Design review of the part built by this model. Coordinates are the model's own, in mm. A direction names the side the tool comes from. Round coordinates to 2 decimals unless told otherwise and drop trailing zeros. Write each loop counter-clockwise with the first axis right and the second up, starting at its lowest first coordinate (ties: lowest second). Pieces come first, ordered by that corner, then holes. Notation, with made-up numbers: (68.5, 57) -> (84.5, 57) arc R16 cw to (84.5, 82) -> close; hole circle Ø4 at (24.25, -21). An arc over 180 degrees is marked (long way). Write item = value, one per line. Start each with the question number.
Item 1: Machinability: for faces 4 (the flat face through (12, 5.359, 0)), 5 (the flat face through (1, 14.275, 3)), 6 (the flat face through (11.836, 6, 0)), which of the approach directions +Z, -Z, +X, -X, +Y, -Y give a long, thin tool a straight path to every point of the face, cutting with its end or side? Answer none if there is none.
Item 2: To check wall thickness, follow L1, parallel to Z at x = 12.5, y = 5.5; L2, parallel to Y at x = 7, z = -2.5; L3, parallel to X at y = 4.75, z = 4.25. State the ranges of each line that lie inside material, in increasing order.
Item 3: Add section D-D, the plane y = 15.5. State the section outline as (x, z) points, then the cut area to 3 significant figures.
Item 4: Add section B-B, the plane z = 0. State the section outline as (x, y) points, then the cut area to 3 significant figures.
Item 5: Mouldability with a two-part tool opening along Z and no side actions: class faces 1 (the flat face through (14, 5.613, 0)), 2 (the flat face through (0, 16.027, 0)), 3 (the cylindrical face through (5.16, 7.58, -1.63)) as released by +Z, released by -Z, zero draft, split by the parting line, or undercut.
Item 6: Add section A-A, the plane x = 10.5. State the section outline as (y, z) points, then the cut area to 3 significant figures.
Item 7: Add section C-C, the plane y = 4. State the section outline as (x, z) points, then the cut area to 3 significant figures.
Item 8: For pin 1 Ø5 at (x, z) = (12, -1.5) entering from +Y; pin 2 Ø2 at (y, z) = (13, 5.5) entering from +X; pin 3 Ø5 at (y, z) = (3.5, 3.5) entering from -X; pin 4 Ø1.1 at (x, z) = (13.5, 6) entering from -Y, all flat-tipped, find the tip position at first contact; note any pin that passes through.
from build123d import *

# Parameters (mm, degrees)
SKETCH1_R           = 8.1534
BOSS_EXTRUDE1_DEPTH = 5.6134
BOSS_EXTRUDE2_DEPTH = 1.27
BOSS_EXTRUDE3_DEPTH = 0.254
SKETCH4_R           = 5.4102
BOSS_EXTRUDE4_DEPTH = 0.889
SKETCH5_R           = 3.3655
BOSS_EXTRUDE5_DEPTH = 6.2484
SKETCH6_R           = 2.9591
BOSS_EXTRUDE6_DEPTH = 8.509
SKETCH7_W           = 8.77263503
SKETCH7_H           = 1.27
CUT_EXTRUDE1_DEPTH  = 6.7564
BOSS_EXTRUDE7_DEPTH = 0.254
LPATTERN1_COUNT     = 2
LPATTERN1_PITCH     = 5.207
LPATTERN2_COUNT     = 2
LPATTERN2_PITCH     = 5.207
FILLET1_R           = 0.762


with BuildPart() as part:
    # Sketch1 → Boss-Extrude1 (new body)
    with BuildSketch(Plane(origin=(0, 0, 0), x_dir=(1, 0, 0), z_dir=(0, 1, 0))):
        Circle(SKETCH1_R)
    extrude(amount=BOSS_EXTRUDE1_DEPTH)

    # Sketch2 → Boss-Extrude2 (add)
    with BuildSketch(Plane(origin=(0, 5.6134, 0), x_dir=(1, 0, 0), z_dir=(0, 1, 0))):
        with BuildLine():
            Line((0, 8.1534), (11.8364, 8.1534))
            Line((11.8364, 8.1534), (11.8364, -8.1534))
            Line((11.8364, -8.1534), (0, -8.1534))
            ThreePointArc((0, -8.1534), (-8.1534, 0), (0, 8.1534))
        make_face()
    extrude(amount=BOSS_EXTRUDE2_DEPTH)

    # Sketch3 → Boss-Extrude3 (add)
    with BuildSketch(Plane(origin=(0, 6.8834, 0), x_dir=(1, 0, 0), z_dir=(0, 1, 0))):
        with BuildLine():
            Line((-5.4737, 5.301227057), (-5.4737, -5.301227057))
            ThreePointArc((-5.4737, -5.301227057), (0, -7.62), (5.4737, -5.301227057))
            Line((5.4737, -5.301227057), (5.4737, 5.301227057))
            ThreePointArc((5.4737, 5.301227057), (0, 7.62), (-5.4737, 5.301227057))
        make_face()
    extrude(amount=BOSS_EXTRUDE3_DEPTH)

    # Sketch4 → Boss-Extrude4 (add)
    with BuildSketch(Plane(origin=(0, 7.1374, 0), x_dir=(1, 0, 0), z_dir=(0, 1, 0))):
        Circle(SKETCH4_R)
    extrude(amount=BOSS_EXTRUDE4_DEPTH)

    # Sketch5 → Boss-Extrude5 (add)
    with BuildSketch(Plane(origin=(0, 8.0264, 0), x_dir=(1, 0, 0), z_dir=(0, 1, 0))):
        Circle(SKETCH5_R)
    extrude(amount=BOSS_EXTRUDE5_DEPTH)

    # Sketch6 → Boss-Extrude6 (add)
    with BuildSketch(Plane(origin=(0, 14.2748, 0), x_dir=(1, 0, 0), z_dir=(0, 1, 0))):
        Circle(SKETCH6_R)
    extrude(amount=BOSS_EXTRUDE6_DEPTH)

    # Sketch7 → Cut-Extrude1 (cut)
    with BuildSketch(Plane(origin=(0, 22.7838, 0), x_dir=(1, 0, 0), z_dir=(0, 1, 0))):
        Rectangle(SKETCH7_W, SKETCH7_H)
    extrude(amount=-CUT_EXTRUDE1_DEPTH, mode=Mode.SUBTRACT)

    # Sketch8 → Boss-Extrude7 (add)
    with BuildSketch(Plane.XZ.offset(-5.6134)):
        Polygon((8.350699667, 1.7526), (12.8524, 1.7526), (12.8524, 0.4826), (16.5862, 0.4826), (16.5862, -0.4826), (12.8524, -0.4826), (12.8524, -1.7526), (8.350699667, -1.7526), align=None)
    boss_extrude7 = extrude(amount=BOSS_EXTRUDE7_DEPTH)

    # LPattern1: Boss-Extrude7 ×2
    with Locations(*[(0, 0, -i * LPATTERN1_PITCH) for i in range(1, LPATTERN1_COUNT)]):
        add(boss_extrude7)

    # LPattern2: Boss-Extrude7 ×2
    with Locations(*[(0, 0, i * LPATTERN2_PITCH) for i in range(1, LPATTERN2_COUNT)]):
        add(boss_extrude7)

    # Fillet1
    fillet1_edges = [part.edges().sort_by_distance(p)[0] for p in [
        (-8.1534, 0, 0),
    ]]
    fillet(fillet1_edges, radius=FILLET1_R)


solid = part.part
Result set:
q1.face_4 = +Z, -Z, +X, -Y
q1.face_5 = +Y
q1.face_6 = +Z, -Z, +X, +Y
q2.L1 = -6.96 to -3.45, -1.75 to 1.75, 3.45 to 6.96
q2.L2 = 0 to 6.88
q2.L3 = -6.96 to 6.96
q3.outline = circle Ø5.92 at (0, 0)
q3.area = 27.5 mm²
q4.outline = (-8.15, 0.76) arc R0.76 ccw to (-7.39, 0) -> (7.39, 0) arc R0.76 ccw to (8.15, 0.76) -> (8.15, 5.61) -> (8.35, 5.61) -> (8.35, 5.36) -> (16.59, 5.36) -> (16.59, 5.61) -> (11.84, 5.61) -> (11.84, 6.88) -> (5.47, 6.88) -> (5.47, 7.14) -> (5.41, 7.14) -> (5.41, 8.03) -> (3.37, 8.03) -> (3.37, 14.27) -> (2.96, 14.27) -> (2.96, 16.03) -> (-2.96, 16.03) -> (-2.96, 14.27) -> (-3.37, 14.27) -> (-3.37, 8.03) -> (-5.41, 8.03) -> (-5.41, 7.14) -> (-5.47, 7.14) -> (-5.47, 6.88) -> (-8.15, 6.88) -> close
q4.area = 184 mm²
q5.face_1 = zero draft
q5.face_2 = undercut
q5.face_3 = split by the parting line
q6.outline = (5.36, -6.96) -> (5.61, -6.96) -> (5.61, -8.15) -> (6.88, -8.15) -> (6.88, 8.15) -> (5.61, 8.15) -> (5.61, 6.96) -> (5.36, 6.96) -> (5.36, 3.45) -> (5.61, 3.45) -> (5.61, 1.75) -> (5.36, 1.75) -> (5.36, -1.75) -> (5.61, -1.75) -> (5.61, -3.45) -> (5.36, -3.45) -> close
q6.area = 23.4 mm²
q7.outline = circle Ø16.31 at (0, 0)
q7.area = 209 mm²
q8.pin_1 = 6.88
q8.pin_2 = through
q8.pin_3 = -8.09
q8.pin_4 = 5.36
